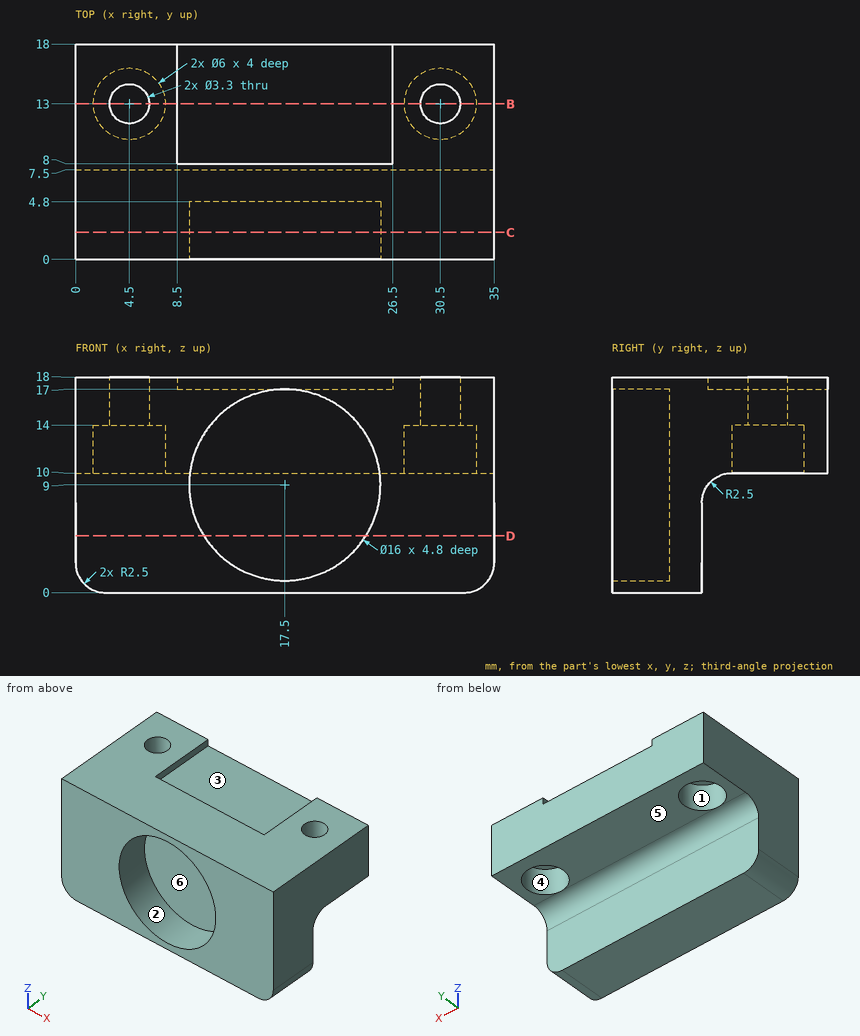
The drawing under review shows one solid part. Ordinate dimensions are in mm from its lowest x, y, z. A direction names the side the tool comes from. Round coordinates to 2 decimals unless told otherwise and drop trailing zeros. Write each loop counter-clockwise with the first axis right and the second up, starting at its lowest first coordinate (ties: lowest second). Pieces come first, ordered by that corner, then holes.
(1) We need section C-C on y = 2.25. Give the boundary of the cut face in (x, z).
(2) We need section D-D on z = 4.75. Give the boundary of the cut face in (x, y), and give its area (3 significant figures).
(3) Mouldability with a two-part tool opening along Z and no side actions: class the marked faces 1, 2 and 3 as +Z half, -Z half, draft (parallel to the pull), parting line (faces both ways), or undercut.
(4) Insertion check: pin 1 (1 mm diameter, centred on x = 22.5, z = 5.5, fed in from -Y); pin 2 (4 mm diameter, centred on x = 4.5, y = 13, fed in from -Z); pin 3 (6.5 mm diameter, centred on x = 29.5, y = 13, fed in from -Z). Each pin has a flat end and moves straight along its axis. Give the tip position at first contact, or say it passes through.
(5) Wall thickness on L1, parallel to X at y = 3.1, z = 9; L2, parallel to Y at x = 30.5, z = 11.75; L3, parallel to Y at x = 2, z = 11.25: over which ranges is each line inside the solid? List them lowest first.
(6) Machinability: for the marked faces 4, 5 and 6, which of the approach directions +Z, -Z, +X, -X, +Y, -Y give a long, thin tool a straight path to every point of the face, cutting with its end or side? Answer none if there is none.
(7) We need section B-B on y = 13. Give the boundary of the cut face in (x, z).
Findings below:
1. outline: (0, 2.5) arc R2.5 ccw to (2.5, 0) - (32.5, 0) arc R2.5 ccw to (35, 2.5) - (35, 18) - (0, 18) - close; hole circle Ø16 at (17.5, 9)
2. outline: (0, 0) - (10.72, 0) - (10.72, 4.8) - (24.28, 4.8) - (24.28, 0) - (35, 0) - (35, 7.5) - (0, 7.5) - close
2. area: 197 mm2
3. face 1: draft
3. face 2: undercut
3. face 3: +Z half
4. pin 1: stops at y = 4.8
4. pin 2: stops at z = 14
4. pin 3: stops at z = 9.99
5. L1: x = 0 to 9.5, 25.5 to 35
5. L2: y = 0 to 10, 16 to 18
5. L3: y = 0 to 11.34, 14.66 to 18
6. face 4: -Z
6. face 5: -Z, +X, -X, +Y
6. face 6: -Y
7. outline: (0, 10) - (1.5, 10) - (1.5, 14) - (2.85, 14) - (2.85, 18) - (0, 18) - close; (6.15, 14) - (7.5, 14) - (7.5, 10) - (27.5, 10) - (27.5, 14) - (28.85, 14) - (28.85, 18) - (26.5, 18) - (26.5, 17) - (8.5, 17) - (8.5, 18) - (6.15, 18) - close; (32.15, 14) - (33.5, 14) - (33.5, 10) - (35, 10) - (35, 18) - (32.15, 18) - close
